CAD build for the part. Positions are in the model's coordinates, mm. Give positions to 0.01 mm unless a question says otherwise; leave off trailing zeros. Loops run counter-clockwise (first coordinate to the right, second up) from the corner with the lowest first, then second, coordinate; pieces in that order, holes last.
Item 1: Saw through at C-C on y = 1.65. Give the cut face in (x, z), plus the area to 3 significant figures.
Item 2: Saw through at A-A on z = 13.5. Give the cut face in (x, y).
Item 3: Probe probe 1 along X at (y, z) = (-1.95, 16.5); probe 2 along X at (y, z) = (1.9, -8.5); probe 3 along Y at (x, z) = (0.1, 0.5). List the from-to ranges inside material, lowest first.
Item 4: Saw through at B-B on x = 1.5. Give the cut face in (y, z).
from build123d import *

# Parameters (mm, degrees)
SKETCH1_R           = 1.5
EXTRUDE1_DEPTH      = 18.5
EXTRUDE1_DEPTH_BACK = 18.5


with BuildPart() as part:
    # Sketch1 → Extrude1 (new, two sides)
    with BuildSketch(Plane.XY) as extrude1_sk:
        Polygon((2.25, -1.299038106), (2.25, 1.299038106), (0, 2.598076211), (-2.25, 1.299038106), (-2.25, -1.299038106), (0, -2.598076211), align=None)
        Circle(SKETCH1_R, mode=Mode.SUBTRACT)
        Circle(SKETCH1_R)
    extrude(amount=EXTRUDE1_DEPTH)
    extrude(extrude1_sk.sketch, amount=-EXTRUDE1_DEPTH_BACK)


solid = part.part
Results below:
1. outline: (-1.64, -18.5) - (1.64, -18.5) - (1.64, 18.5) - (-1.64, 18.5) - close
1. area: 122 mm2
2. outline: (-2.25, -1.3) - (0, -2.6) - (2.25, -1.3) - (2.25, 1.3) - (0, 2.6) - (-2.25, 1.3) - close
3. probe 1: x = -1.12 to 1.12
3. probe 2: x = -1.21 to 1.21
3. probe 3: y = -2.54 to 2.54
4. outline: (-1.73, -18.5) - (1.73, -18.5) - (1.73, 18.5) - (-1.73, 18.5) - close
